The model under review builds one solid part; all positions refer to its coordinate system, in mm. A direction names the side the tool comes from. Round coordinates to 2 decimals unless told otherwise and drop trailing zeros. Write each loop counter-clockwise with the first axis right and the second up, starting at its lowest first coordinate (ties: lowest second). Pieces come first, ordered by that corner, then holes. Notation, with made-up numbers: (10.25, 31.5) - (20.25, 31.5) arc R33 ccw to (20.25, 69.5) - close; hole circle Ø3 at (-28, 80). An arc over 180 degrees is marked (long way). Use one line per item in the form item = value.
from build123d import *

# Parameters (mm, degrees)
SALIENTE_EXTRUIR1_DEPTH    = 131.1
CROQUIS3_R                 = 1.1
CORTAR_EXTRUIR1_DEPTH      = 289.575068223
CROQUIS4_R                 = 10.7
CROQUIS4_R_2               = 5.07
CROQUIS4_W                 = 121.1
CROQUIS4_H                 = 75.8
CROQUIS4_W_2               = 1.6
CROQUIS4_H_2               = 10
CROQUIS4_W_3               = 10
CROQUIS4_H_3               = 10.6
CORTAR_EXTRUIR2_DEPTH      = 287.189954401
CROQUIS7_W                 = 1.36
CROQUIS7_H                 = 98
CROQUIS7_W_2               = 1.86
CROQUIS7_H_2               = 41.6
SALIENTE_EXTRUIR2_DEPTH    = 4.4
CROQUIS8_R                 = 2.27
CORTAR_EXTRUIR3_DEPTH      = 1.8
CORTAR_EXTRUIR4_START      = -1.8
CROQUIS9_R                 = 2.27
CORTAR_EXTRUIR4_DEPTH      = 1.8
CROQUIS10_R                = 11.9
CROQUIS10_R_2              = 10.7
CROQUIS10_W                = 12.4
CROQUIS10_H                = 13
CROQUIS10_W_2              = 10
CROQUIS10_H_2              = 10.6
SALIENTE_EXTRUIR4_DEPTH    = 8.6
REDONDEO2_R                = 1.28
CORTAR_EXTRUIR5_REACH      = 292.482
CORTAR_EXTRUIR5_END_RADIUS = 10.7
CROQUIS11_W                = 4
CROQUIS11_H                = 14
SALIENTE_EXTRUIR6_START    = 1
CROQUIS13_W                = 12.4
CROQUIS13_H                = 13
SALIENTE_EXTRUIR6_DEPTH    = 1
CROQUIS14_R                = 2.8
CROQUIS14_R_2              = 1.5
SALIENTE_EXTRUIR7_DEPTH    = 8.4
REDONDEO3_R                = 1.28
CROQUIS17_W                = 4.4
CROQUIS17_H                = 0.4
CORTAR_EXTRUIR6_DEPTH      = 285.106479335
REDONDEO4_R                = 1.6
CROQUIS19_R                = 1.12
SALIENTE_EXTRUIR8_DEPTH    = 8.6
REDONDEO5_R                = 1
CORTAR_EXTRUIR8_START      = -1.86
CROQUIS21_W                = 0.6
CROQUIS21_H                = 26
CORTAR_EXTRUIR8_DEPTH      = 1.86
CROQUIS23_W                = 121.1
CROQUIS23_H                = 0.1
CORTAR_EXTRUIR9_DEPTH      = 287.189954401


with BuildPart() as part:
    # Croquis2 → Saliente-Extruir1 (new body)
    with BuildSketch(Plane(origin=(0, 0, 0), x_dir=(0, 0, -1), z_dir=(1, 0, 0))):
        with BuildLine():
            Line((37, 0), (37, -3.2))
            Line((37, -3.2), (8.4, -3.2))
            ThreePointArc((8.4, -3.2), (0.197561338, 0.197561338), (-3.2, 8.4))
            Line((-3.2, 8.4), (-3.2, 239.6))
            ThreePointArc((-3.2, 239.6), (0.197561338, 247.802438662), (8.4, 251.2))
            Line((8.4, 251.2), (37, 251.2))
            Line((37, 251.2), (37, 248))
            Line((37, 248), (8.4, 248))
            ThreePointArc((8.4, 248), (2.460303038, 245.539696962), (0, 239.6))
            Line((0, 239.6), (0, 8.4))
            ThreePointArc((0, 8.4), (2.460303038, 2.460303038), (8.4, 0))
            Line((8.4, 0), (37, 0))
        make_face()
    extrude(amount=SALIENTE_EXTRUIR1_DEPTH)

    # Croquis3 → Cortar-Extruir1 (cut, through all)
    with BuildSketch(Plane(origin=(0, 251.2, 0), x_dir=(1, 0, 0), z_dir=(0, 1, 0))):
        with Locations(Location((6.55, 22.7, 0), (0, 0, 270))):
            Circle(CROQUIS3_R)
        with Locations(Location((124.55, 22.7, 0), (0, 0, 270))):
            Circle(CROQUIS3_R)
    extrude(amount=-CORTAR_EXTRUIR1_DEPTH, mode=Mode.SUBTRACT)

    # Croquis4 → Cortar-Extruir2 (cut, through all)
    with BuildSketch(Plane.XY.offset(3.2)):
        with Locations((17, 78.7)):
            Circle(CROQUIS4_R)
        with Locations((65.55, 113.5)):
            Circle(CROQUIS4_R_2)
        with Locations((65.55, 196.1)):
            Rectangle(CROQUIS4_W, CROQUIS4_H)
        with Locations((9.2, 112)):
            Rectangle(CROQUIS4_W_2, CROQUIS4_H_2)
        with Locations((46.5, 91.4)):
            Rectangle(CROQUIS4_W_3, CROQUIS4_H_3)
        with Locations((5.8, 112)):
            Rectangle(CROQUIS4_W_2, CROQUIS4_H_2)
        with Locations((12.6, 112)):
            Rectangle(CROQUIS4_W_2, CROQUIS4_H_2)
        with Locations((16, 112)):
            Rectangle(CROQUIS4_W_2, CROQUIS4_H_2)
        with Locations((19.4, 112)):
            Rectangle(CROQUIS4_W_2, CROQUIS4_H_2)
        with Locations((22.8, 112)):
            Rectangle(CROQUIS4_W_2, CROQUIS4_H_2)
        with Locations((26.2, 112)):
            Rectangle(CROQUIS4_W_2, CROQUIS4_H_2)
        with Locations((29.6, 112)):
            Rectangle(CROQUIS4_W_2, CROQUIS4_H_2)
        with Locations((33, 112)):
            Rectangle(CROQUIS4_W_2, CROQUIS4_H_2)
        with Locations((36.4, 112)):
            Rectangle(CROQUIS4_W_2, CROQUIS4_H_2)
        with Locations((39.8, 112)):
            Rectangle(CROQUIS4_W_2, CROQUIS4_H_2)
        with Locations((43.2, 112)):
            Rectangle(CROQUIS4_W_2, CROQUIS4_H_2)
        with Locations((46.6, 112)):
            Rectangle(CROQUIS4_W_2, CROQUIS4_H_2)
        with Locations((50, 112)):
            Rectangle(CROQUIS4_W_2, CROQUIS4_H_2)
    extrude(amount=-CORTAR_EXTRUIR2_DEPTH, mode=Mode.SUBTRACT)

    # Croquis7 → Saliente-Extruir2 (add)
    with BuildSketch(Plane(origin=(0, 0, 0), x_dir=(-1, 0, 0), z_dir=(0, 0, -1))):
        Polygon((-127.46, 125.3), (-127.96, 125.3), (-127.96, 66.3), (-127.46, 66.3), (-126.1, 66.3), (-126.1, 125.3), align=None)
        with Locations((-126.78, 185)):
            Rectangle(CROQUIS7_W, CROQUIS7_H)
        with Locations((-4.32, 185)):
            Rectangle(CROQUIS7_W, CROQUIS7_H)
        Polygon((-3.64, 125.3), (-5, 125.3), (-5, 66.3), (-3.64, 66.3), (-3.14, 66.3), (-3.14, 125.3), align=None)
        with Locations((-127.03, 32.7)):
            Rectangle(CROQUIS7_W_2, CROQUIS7_H_2)
        with Locations((-4.07, 32.7)):
            Rectangle(CROQUIS7_W_2, CROQUIS7_H_2)
    extrude(amount=SALIENTE_EXTRUIR2_DEPTH)

    # Croquis8 → Cortar-Extruir3 (cut)
    with BuildSketch(Plane(origin=(0, 251.2, 0), x_dir=(1, 0, 0), z_dir=(0, 1, 0))):
        with Locations(Location((6.55, 22.7, 0), (0, 0, 270))):
            Circle(CROQUIS8_R)
        with Locations(Location((124.55, 22.7, 0), (0, 0, 270))):
            Circle(CROQUIS8_R)
    extrude(amount=-CORTAR_EXTRUIR3_DEPTH, mode=Mode.SUBTRACT)

    # Croquis9 → Cortar-Extruir4 (cut)
    with BuildSketch(Plane.XZ.offset(3.2).offset(CORTAR_EXTRUIR4_START)):
        with Locations(Location((124.55, -22.7, 0), (0, 0, 90))):
            Circle(CROQUIS9_R)
        with Locations(Location((6.55, -22.7, 0), (0, 0, 90))):
            Circle(CROQUIS9_R)
    extrude(amount=CORTAR_EXTRUIR4_DEPTH, mode=Mode.SUBTRACT)

    # Croquis10 → Saliente-Extruir4 (add)
    # profile 1 of 2: a face of its own
    with BuildSketch(Plane(origin=(0, 0, 0), x_dir=(-1, 0, 0), z_dir=(0, 0, -1))):
        with Locations(Location((-17, 78.7, 0), (0, 0, 180))):
            Circle(CROQUIS10_R)
        with Locations(Location((-17, 78.7, 0), (0, 0, 180))):
            Circle(CROQUIS10_R_2, mode=Mode.SUBTRACT)
    # profile 2 of 2: a face of its own
    with BuildSketch(Plane(origin=(0, 0, 0), x_dir=(-1, 0, 0), z_dir=(0, 0, -1))):
        with Locations((-46.5, 91.4)):
            Rectangle(CROQUIS10_W, CROQUIS10_H)
        with Locations((-46.5, 91.4)):
            Rectangle(CROQUIS10_W_2, CROQUIS10_H_2, mode=Mode.SUBTRACT)
    extrude(amount=SALIENTE_EXTRUIR4_DEPTH)

    # Redondeo2
    redondeo2_edges = [part.edges().sort_by_distance(p)[0] for p in [
        (41.5, 86.1, -2.7),
        (41.5, 96.7, -2.7),
        (51.5, 96.7, -2.7),
        (51.5, 86.1, -2.7),
    ]]
    fillet(redondeo2_edges, radius=REDONDEO2_R)

    # Cortar-Extruir5: up to this cylinder (the profile starts outside it)
    cortar_extruir5_end = Plane(origin=(17, 78.7, -4.3), z_dir=(0, 0, 1)) * Cylinder(CORTAR_EXTRUIR5_END_RADIUS, 607.364, mode=Mode.PRIVATE)
    # Croquis11 → Cortar-Extruir5 (cut, up to the surface)
    with BuildSketch(Plane.ZY.offset(10), mode=Mode.PRIVATE) as cortar_extruir5_sk1:
        with Locations((-4.3, 78.7)):
            Rectangle(CROQUIS11_W, CROQUIS11_H)
    cortar_extruir5_tool1 = extrude(cortar_extruir5_sk1.sketch, amount=-CORTAR_EXTRUIR5_REACH, mode=Mode.PRIVATE) - cortar_extruir5_end
    add(cortar_extruir5_tool1.solids().sort_by_distance((-10, 78.7, -4.3))[0], mode=Mode.SUBTRACT)

    # Croquis13 → Saliente-Extruir6 (add)
    with BuildSketch(Plane(origin=(0, 0, -8.6), x_dir=(-1, 0, 0), z_dir=(0, 0, -1)).offset(SALIENTE_EXTRUIR6_START)):
        with Locations((-46.5, 91.4)):
            Rectangle(CROQUIS13_W, CROQUIS13_H)
        with BuildLine():
            ThreePointArc((-50.22, 86.1), (-51.12509668, 86.47490332), (-51.5, 87.38))
            Line((-51.5, 87.38), (-51.5, 95.42))
            ThreePointArc((-51.5, 95.42), (-51.12509668, 96.32509668), (-50.22, 96.7))
            Line((-50.22, 96.7), (-42.78, 96.7))
            ThreePointArc((-42.78, 96.7), (-41.87490332, 96.32509668), (-41.5, 95.42))
            Line((-41.5, 95.42), (-41.5, 87.38))
            ThreePointArc((-41.5, 87.38), (-41.87490332, 86.47490332), (-42.78, 86.1))
            Line((-42.78, 86.1), (-50.22, 86.1))
        make_face(mode=Mode.SUBTRACT)
    extrude(amount=-SALIENTE_EXTRUIR6_DEPTH)

    # Croquis14 → Saliente-Extruir7 (add)
    with BuildSketch(Plane(origin=(0, 0, 0), x_dir=(-1, 0, 0), z_dir=(0, 0, -1))):
        with Locations(Location((-65.55, 88.8, 0), (0, 0, 180))):
            Circle(CROQUIS14_R)
        with Locations((-65.55, 88.8)):
            Circle(CROQUIS14_R_2, mode=Mode.SUBTRACT)
    extrude(amount=SALIENTE_EXTRUIR7_DEPTH)

    # Redondeo3
    redondeo3_edges = [part.edges().sort_by_distance(p)[0] for p in [
        (62.75, 88.8, 0),
    ]]
    fillet(redondeo3_edges, radius=REDONDEO3_R)

    # Croquis17 → Cortar-Extruir6 (cut, through all)
    with BuildSketch(Plane(origin=(127.46, 0, 0), x_dir=(0, 0, -1), z_dir=(1, 0, 0))):
        with Locations((2.2, 233.8)):
            Rectangle(CROQUIS17_W, CROQUIS17_H)
    extrude(amount=-CORTAR_EXTRUIR6_DEPTH, mode=Mode.SUBTRACT)

    # Redondeo4
    redondeo4_edges = [part.edges().sort_by_distance(p)[0] for p in [
        (52.7, 91.4, 0),
        (40.3, 91.4, 0),
    ]]
    fillet(redondeo4_edges, radius=REDONDEO4_R)

    # Croquis19 → Saliente-Extruir8 (add)
    with BuildSketch(Plane(origin=(0, 0, 0), x_dir=(-1, 0, 0), z_dir=(0, 0, -1))):
        with Locations((-17, 90.6)):
            Circle(CROQUIS19_R)
        with Locations((-17, 66.8)):
            Circle(CROQUIS19_R)
    extrude(amount=SALIENTE_EXTRUIR8_DEPTH)

    # Redondeo5
    redondeo5_edges = [part.edges().sort_by_distance(p)[0] for p in [
        (28.9, 78.7, 0),
    ]]
    fillet(redondeo5_edges, radius=REDONDEO5_R)

    # Croquis21 → Cortar-Extruir8 (cut)
    with BuildSketch(Plane(origin=(127.96, 0, 0), x_dir=(0, 0, -1), z_dir=(1, 0, 0)).offset(CORTAR_EXTRUIR8_START)):
        with Locations((4.1, 79.3)):
            Rectangle(CROQUIS21_W, CROQUIS21_H)
    extrude(amount=CORTAR_EXTRUIR8_DEPTH, mode=Mode.SUBTRACT)

    # Croquis23 → Cortar-Extruir9 (cut, through all)
    with BuildSketch(Plane.XY.offset(3.2)):
        with Locations((65.55, 158.15)):
            Rectangle(CROQUIS23_W, CROQUIS23_H)
    extrude(amount=-CORTAR_EXTRUIR9_DEPTH, mode=Mode.SUBTRACT)


solid = part.part
(1) Add section B-B on x = 99. Write out the cut boundary in (y, z), then the cut area to 3 significant figures.
Geometry results:
outline = (-3.2, -37) - (0, -37) - (0, -8.4) arc R8.4 cw to (8.4, 0) - (158.1, 0) - (158.1, 3.2) - (8.4, 3.2) arc R11.6 ccw to (-3.2, -8.4) - close; (234, 0) - (239.6, 0) arc R8.4 cw to (248, -8.4) - (248, -37) - (251.2, -37) - (251.2, -8.4) arc R11.6 ccw to (239.6, 3.2) - (234, 3.2) - close
area = 781 mm2
(2) Add section D-D on y = 29.5. Write out the cut boundary in (x, z), then the cut area to 3 significant figures.
Geometry results:
outline = (0, 0) - (3.14, 0) - (3.14, -4.4) - (5, -4.4) - (5, 0) - (126.1, 0) - (126.1, -4.4) - (127.96, -4.4) - (127.96, 0) - (131.1, 0) - (131.1, 3.2) - (0, 3.2) - close
area = 436 mm2
(3) The part is to be moulded in two halves that separate along Z. For faces 4 (the flat face through (41, 91, -9.6)), 5 (the flat face through (6, 249.4, -24)), 6 (the flat face through (41.5, 91, -3)), say which applies: +Z half, -Z half, draft (parallel to the pull), parting line (faces both ways), or undercut.
Geometry results:
face_4 = -Z half
face_5 = undercut
face_6 = draft
(4) Insertion check: P1, Ø1.3, axis at x = 9.5, z = 1, coming from the +Y side; P2, Ø1, axis at x = 88.5, z = 1.5, coming from the -Y side; P3, Ø10, axis at x = 54, y = 154, coming from the -Z side. Each pin has a flat end and moves straight along its axis. Give the tip position at first contact, or say it passes through.
Geometry results:
P1 = 247.22
P2 = 1.6
P3 = 0
(5) To check wall thickness, follow L1, parallel to X at y = -2.1, z = -22.7; L2, parallel to Y at x = 115, z = -28.5; L3, parallel to Y at x = 65.55, z = 1.2. State the ranges of each line that lie inside material, in increasing order.
Geometry results:
L1 = 0 to 4.28, 8.82 to 122.28, 126.82 to 131.1
L2 = -3.2 to 0, 248 to 251.2
L3 = 1.89 to 108.43, 118.57 to 158.1, 234 to 246.11
(6) Machinability: for faces 1 (the flat face through (51.5, 91, -3)), 2 (the flat face through (126.1, 32, -2)), 3 (the flat face through (8, -1.4, -23)), which of the approach directions +Z, -Z, +X, -X, +Y, -Y give a long, thin tool a straight path to every point of the face, cutting with its end or side? Answer none if there is none.
Geometry results:
face_1 = +Z, -Z
face_2 = -Z
face_3 = -Y
(7) Add section C-C on y = 113.5. Count the separate pieces of the cut face and the enclosed holes in it, then the cut area to 3 significant figures.
Geometry results:
separate_pieces = 16
enclosed_holes = 0
area = 332 mm2
(8) Add section A-A on y = 181. Write out the cut boundary in (x, z).
Geometry results:
outline = (0, 0) - (3.64, 0) - (3.64, -4.4) - (5, -4.4) - (5, 3.2) - (0, 3.2) - close; (126.1, -4.4) - (127.46, -4.4) - (127.46, 0) - (131.1, 0) - (131.1, 3.2) - (126.1, 3.2) - close
